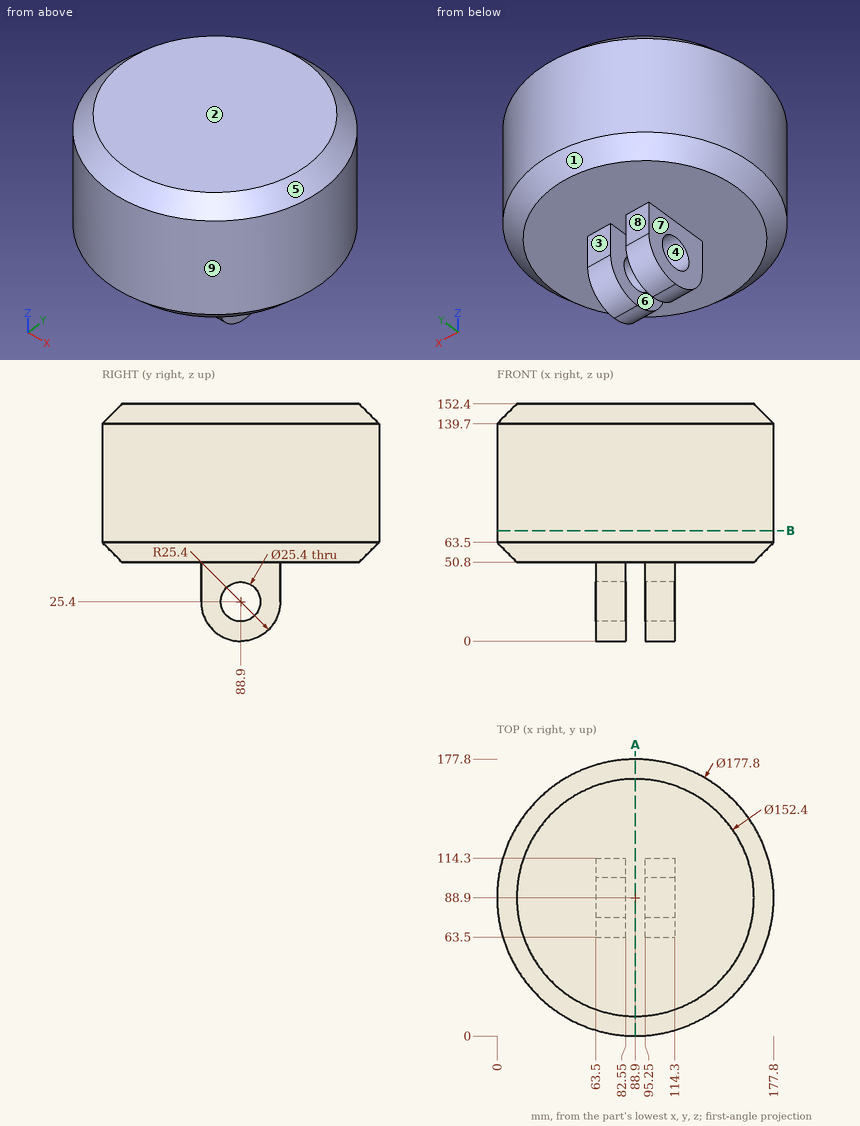
Part print with two shaded views. Sizes in mm from the minimum x, y, z corner. A direction names the side the tool comes from. Round coordinates to 2 decimals unless told otherwise and drop trailing zeros. Order: outer loops, then holes, each group sorted by start corner. A loop starts at its lowest first (then second) coordinate and runs counter-clockwise, first axis right, second up. Notation, with made-up numbers: M -7.75,62.25 L 4.25,62.25 A25 cw 4.25,94.25 Z; hole C 5,4 d3. An arc over 180 degrees is marked long. Put each result on its own line as item: value. Start each with the question number.
1. Drill centre lines: probe 1 along Y at (x, z) = (73, 25); probe 2 along Z at (x, y) = (68, 88.9); probe 3 along Z at (x, y) = (81, 147.5). Where is each one in solid material? Low to high. Write a range as [from, to].
2. Tool access for the marked faces 5, 6, 7, 8 and 9: list every direction of +Z, -Z, +X, -X, +Y, -Y with a clear straight run to the whole face (end or side of a thin tool).
3. Slice it at B-B on z = 71. List the corners of the cut face in (x, y).
4. Two-plate mould, pull along Z, no slides. Class the marked faces 1, 2, 3 and 4: +Z half, -Z half, draft (parallel to the pull), parting line (faces both ways), or undercut.
5. Slice it at A-A on x = 88.9. List the corners of the cut face in (y, z).
6. Drop flat-ended pins along their axis: pin 1 (21 mm diameter, centred on x = 71, z = 42, fed in from +Y); pin 2 (8 mm diameter, centred on x = 109.5, y = 74, fed in from -Z); pin 3 (1.5 mm diameter, centred on y = 47, z = 118.5, fed in from -X). Give the stop position or say it passes through.
Findings:
1. probe 1: [63.5, 76.21], [101.59, 114.3]
1. probe 2: [0, 12.7], [38.1, 152.4]
1. probe 3: [50.8, 152.4]
2. face 5: +Z
2. face 6: -Z, +Y, -Y
2. face 7: -Z, -X, +Y, -Y
2. face 8: -Z, +X, -X, +Y
2. face 9: +Z, -Z
3. outline: C 88.9,88.9 d177.8
4. face 1: -Z half
4. face 2: +Z half
4. face 3: draft
4. face 4: undercut
5. outline: M 0,63.5 L 12.7,50.8 L 165.1,50.8 L 177.8,63.5 L 177.8,139.7 L 165.1,152.4 L 12.7,152.4 L 0,139.7 Z
6. pin 1: y = 164.96
6. pin 2: z = 2.46
6. pin 3: x = 10.1
